```python
from build123d import *

# Parameters (mm, degrees)
F0_R     = 14.1351
F1_DEPTH = 11.303
F2_R     = 0.254
F3_R     = 0.381
F4_DEPTH = 25.4


with BuildPart() as f1:
    # F0 (on Top) → F1 (new body)
    with BuildSketch(Plane.XY):
        Circle(F0_R)
    extrude(amount=F1_DEPTH)

    # F2
    f2_edges = [f1.edges().sort_by_distance(p)[0] for p in [
        (-14.1351, 0, 11.303),
        (-14.1351, 0, 0),
    ]]
    fillet(f2_edges, radius=F2_R)

    # F3 (on face) → F4 (cut)
    with BuildSketch(Plane.XY.offset(11.303)):
        Circle(F3_R)
    extrude(amount=-F4_DEPTH, mode=Mode.SUBTRACT)


solid = f1.part
```
Can you work these out from the model? Positions are in its coordinate system, mm. Coordinates: 2 decimals unless noted, no trailing zeros. Loops run counter-clockwise (first coordinate to the right, second up) from the corner with the lowest first, then second, coordinate; pieces in that order, holes last.
Item 1: Please list where these lines run through material, in increasing order: L1, parallel to Y at x = 0, z = 8.5; L2, parallel to Y at x = 10.25, z = 10.25; L3, parallel to Y at x = 8.5, z = 3.25.
Answers below:
L1: y = -14.14 to -0.38, 0.38 to 14.14
L2: y = -9.73 to 9.73
L3: y = -11.29 to 11.29
Item 2: I'm going to push flat-ended pins straight in: pin 1 (1.5 mm diameter, centred on x = 7.5, z = 4, fed in from -Y); pin 2 (5 mm diameter, centred on x = -6, z = 3.5, fed in from +Y); pin 3 (5 mm diameter, centred on x = -11, z = 9, fed in from +Y); pin 4 (5 mm diameter, centred on x = 4, y = 11, fed in from -Z). Where does each tip first touch, or does it pass through?
Answers below:
pin 1: stops at y = -12.42
pin 2: stops at y = 13.69
pin 3: stops at y = 11.29
pin 4: stops at z = 0
Item 3: Suppose I cut it at A-A (x = 0). Please give me the cut outline in (y, z).
Answers below:
outline: (-14.14, 0.25) arc R0.25 ccw to (-13.88, 0) - (-0.38, 0) - (-0.38, 11.3) - (-13.88, 11.3) arc R0.25 ccw to (-14.14, 11.05) - close; (0.38, 0) - (13.88, 0) arc R0.25 ccw to (14.14, 0.25) - (14.14, 11.05) arc R0.25 ccw to (13.88, 11.3) - (0.38, 11.3) - close
Item 4: Suppose I cut it at C-C (z = 6.25). Please give me the cut outline in (x, y).
Answers below:
outline: circle Ø28.27 at (0, 0); hole circle Ø0.76 at (0, 0)
